```python
from build123d import *

# Parameters (mm, degrees)
SKETCH12_R          = 57.15
SKETCH12_R_2        = 48.641
BOSS_EXTRUDE1_DEPTH = 177.8
CUT_EXTRUDE1_DEPTH  = 196.30766754
CIRPATTERN1_COUNT   = 2
CIRPATTERN1_ANGLE   = 90


with BuildPart() as part:
    # Sketch12 → Boss-Extrude1 (new body)
    with BuildSketch(Plane.XY):
        Circle(SKETCH12_R)
        Circle(SKETCH12_R_2, mode=Mode.SUBTRACT)
    extrude(amount=BOSS_EXTRUDE1_DEPTH)

    # Sketch13 → Cut-Extrude1 (cut, symmetric)
    with BuildSketch(Plane(origin=(0, 0, 0), x_dir=(1, 0, 0), z_dir=(0, 1, 0))):
        with BuildLine():
            Line((-12.7, 0), (12.7, 0))
            Line((12.7, 0), (12.7, -76.2))
            ThreePointArc((12.7, -76.2), (0, -88.9), (-12.7, -76.2))
            Line((-12.7, -76.2), (-12.7, 0))
        make_face()
    cut_extrude1 = extrude(amount=CUT_EXTRUDE1_DEPTH, both=True, mode=Mode.SUBTRACT)

    # CirPattern1: Cut-Extrude1 ×2 about axis
    cirpattern1_axis = Axis((0, 0, 0), (0, 0, 1))
    for i in range(1, CIRPATTERN1_COUNT):
        add(cut_extrude1.rotate(cirpattern1_axis, i * CIRPATTERN1_ANGLE / (CIRPATTERN1_COUNT - 1)), mode=Mode.SUBTRACT)


solid = part.part
```
Could you check a few things on this model? Use its own coordinates, in mm. A direction names the side the tool comes from. Give positions to 0.01 mm unless a question says otherwise; leave off trailing zeros. Order: outer loops, then holes, each group sorted by start corner. A loop starts at its lowest first (then second) coordinate and runs counter-clockwise, first axis right, second up.
Q1. For faces 4 (the flat face through (-51, 12.7, 38)), 5 (the flat face through (12.7, 51, 38)), 6 (the flat face through (36, -37, 0)), which set-ups out of +Z, -Z, +X, -X, +Y, -Y let a thin tool reach every point of the face, with its end or its side?
Q2. Suppose I cut it at A-A, the plane y = 0. Write out the boundary of the cut face in (x, z).
Q3. I'm going to push flat-ended pins straight in: P1, Ø7, axis at x = 52, z = 25, coming from the -Y side; P2, Ø12, axis at x = 40, z = 106, coming from the -Y side; P3, Ø2.5, axis at y = 51.5, z = 29, coming from the +X side. Where does each tip first touch, or does it pass through?
Q4. Suppose I cut it at D-D, the plane z = 123.5. Write out the boundary of the cut face in (x, y), and give its area (3 significant figures).
Q5. Suppose I cut it at C-C, the plane z = 30. Write out the boundary of the cut face in (x, y).
Q6. We'd pull the mould along Y, two halves only. Please class faces 1 (the flat face through (-12.7, -51, 39)), 2 (the flat face through (-51, -12.7, 39)), 3 (the cylindrical face through (54.5, 17.2, 87.7)): +Y half, -Y half, draft (parallel to the pull), parting line (faces both ways), or undercut.
Q7. If I drill on line 1 along Y through (x, z) = (0, 122); line 2 along Y through (x, z) = (-45, 29), over which ranges is the centre line in solid material (lowest first)?
Solution:
1. face 4: -Z, +X, -X
1. face 5: -Z, +Y, -Y
1. face 6: -Z, +X, -X, +Y, -Y
2. outline: (-57.15, 88.9) - (-48.64, 88.9) - (-48.64, 177.8) - (-57.15, 177.8) - close; (48.64, 88.9) - (57.15, 88.9) - (57.15, 177.8) - (48.64, 177.8) - close
3. P1: stops at y = -30.23
3. P2: stops at y = -45.94
3. P3: stops at x = 27.22
4. outline: circle Ø114.3 at (0, 0); hole circle Ø97.28 at (0, 0)
4. area: 2,830 mm2
5. outline: (-55.72, -12.7) arc R57.15 ccw to (-12.7, -55.72) - (-12.7, -46.95) arc R48.64 cw to (-46.95, -12.7) - close; (-55.72, 12.7) - (-46.95, 12.7) arc R48.64 cw to (-12.7, 46.95) - (-12.7, 55.72) arc R57.15 ccw to start; (12.7, -55.72) arc R57.15 ccw to (55.72, -12.7) - (46.95, -12.7) arc R48.64 cw to (12.7, -46.95) - close; (12.7, 46.95) arc R48.64 cw to (46.95, 12.7) - (55.72, 12.7) arc R57.15 ccw to (12.7, 55.72) - close
6. face 1: draft
6. face 2: undercut
6. face 3: parting line
7. line 1: y = -57.15 to -48.64, 48.64 to 57.15
7. line 2: y = -35.23 to -18.46, 18.46 to 35.23
